CAD build for the part. Positions are in the model's coordinates, mm. A direction names the side the tool comes from. Give positions to 0.01 mm unless a question says otherwise; leave off trailing zeros. Loops run counter-clockwise (first coordinate to the right, second up) from the corner with the lowest first, then second, coordinate; pieces in that order, holes last.
Item 1: Saw through at C-C on y = -5.5. Give the cut face in (x, z).
Item 2: Probe probe 1 along Y at (x, z) = (7.5, 6.25); probe 2 along Y at (x, z) = (-22, 4.5); probe 3 along Z at (x, y) = (16, -16.5). List the from-to ranges inside material, lowest first.
Item 3: Which spindle directions (+Z, -Z, +X, -X, +Y, -Y) get a long thin tool onto all of the face, cutting with end or side? Do faces 4 (the flat face through (0, -16.25, 5)), 5 (the flat face through (0, 16, 7)). Say none if no direction does.
Item 4: Saw through at B-B on x = 15.5. Give the cut face in (y, z), plus the area to 4 significant figures.
Item 5: Drop flat-ended pins along their axis: P1, Ø1.5, axis at x = 11.5, y = -20, coming from the +Z side; P2, Ø4, axis at y = -17, z = 5, coming from the +X side. Give the stop position or say it passes through.
Item 6: Saw through at D-D on z = 2.5. Give the cut face in (x, y).
Item 7: Saw through at A-A on z = 6.25. Give the cut face in (x, y).
Item 8: Mould opens along Y. For faces 1 (the flat face through (0, -21.25, 5)), 2 (the flat face through (0, -28.75, 3)), 3 (the flat face through (0, -14, 7)) say: released by +Y, released by -Y, zero draft, split by the parting line, or undercut.
from build123d import *

# Parameters (mm, degrees)
EXTRUDE1_DEPTH = 4
EXTRUDE2_DEPTH = 3


with BuildPart() as part:
    # Sketch1 → Extrude1 (new body)
    with BuildSketch(Plane.XY):
        Polygon((-25.1, -28.75), (-16.5, 28.75), (16.5, 28.75), (25.1, -28.75), align=None)
    extrude(amount=EXTRUDE1_DEPTH)

    # Sketch2 → Extrude2 (add)
    with BuildSketch(Plane.XY.offset(4)):
        Polygon((-17.247826087, 23.75), (17.247826087, 23.75), (16.5, 28.75), (-16.5, 28.75), align=None)
        Polygon((-17.995652174, 18.75), (17.995652174, 18.75), (18.743478261, 13.75), (-18.743478261, 13.75), align=None)
        Polygon((-19.491304348, 8.75), (19.491304348, 8.75), (20.239130435, 3.75), (-20.239130435, 3.75), align=None)
        Polygon((-25.1, -28.75), (25.1, -28.75), (23.97826087, -21.25), (-23.97826087, -21.25), align=None)
        Polygon((-20.986956522, -1.25), (20.986956522, -1.25), (21.734782609, -6.25), (-21.734782609, -6.25), align=None)
        Polygon((-22.482608696, -11.25), (22.482608696, -11.25), (23.230434783, -16.25), (-23.230434783, -16.25), align=None)
    extrude(amount=EXTRUDE2_DEPTH)


solid = part.part
Results below:
1. outline: (-21.62, 0) - (21.62, 0) - (21.62, 7) - (-21.62, 7) - close
2. probe 1: y = -28.75 to -21.25, -16.25 to -11.25, -6.25 to -1.25, 3.75 to 8.75, 13.75 to 18.75, 23.75 to 28.75
2. probe 2: y = -28.75 to -21.25, -16.25 to -11.25
2. probe 3: z = 0 to 4
3. face 4: +Z, +X, -X
3. face 5: +Z, +X, -X, +Y, -Y
4. outline: (-28.75, 0) - (28.75, 0) - (28.75, 7) - (23.75, 7) - (23.75, 4) - (18.75, 4) - (18.75, 7) - (13.75, 7) - (13.75, 4) - (8.75, 4) - (8.75, 7) - (3.75, 7) - (3.75, 4) - (-1.25, 4) - (-1.25, 7) - (-6.25, 7) - (-6.25, 4) - (-11.25, 4) - (-11.25, 7) - (-16.25, 7) - (-16.25, 4) - (-21.25, 4) - (-21.25, 7) - (-28.75, 7) - close
4. area: 327.5 mm2
5. P1: stops at z = 4
5. P2: stops at x = 23.6
6. outline: (-25.1, -28.75) - (25.1, -28.75) - (16.5, 28.75) - (-16.5, 28.75) - close
7. outline: (-25.1, -28.75) - (25.1, -28.75) - (23.98, -21.25) - (-23.98, -21.25) - close; (-23.23, -16.25) - (23.23, -16.25) - (22.48, -11.25) - (-22.48, -11.25) - close; (-21.73, -6.25) - (21.73, -6.25) - (20.99, -1.25) - (-20.99, -1.25) - close; (-20.24, 3.75) - (20.24, 3.75) - (19.49, 8.75) - (-19.49, 8.75) - close; (-18.74, 13.75) - (18.74, 13.75) - (18, 18.75) - (-18, 18.75) - close; (-17.25, 23.75) - (17.25, 23.75) - (16.5, 28.75) - (-16.5, 28.75) - close
8. face 1: undercut
8. face 2: released by -Y
8. face 3: zero draft
